from build123d import *

# Parameters (mm, degrees)
SKETCH1_W               = 49.5
SKETCH1_H               = 61.5
BOSS_EXTRUDE1_DEPTH     = 23.75
SKETCH2_W               = 46
SKETCH2_H               = 58
CUT_EXTRUDE1_DEPTH      = 22
SKETCH3_W               = 3
SKETCH3_H               = 16
CUT_EXTRUDE2_DEPTH      = 1.75
SKETCH7_W               = 3
SKETCH7_H               = 5
BOSS_EXTRUDE2_DEPTH     = 4
SKETCH11_W              = 37.5
SKETCH11_H              = 61.5
BOSS_EXTRUDE3_DEPTH     = 15
SKETCH12_W              = 34
SKETCH12_H              = 57
CUT_EXTRUDE3_DEPTH      = 15
SKETCH14_W              = 7.75
SKETCH14_H              = 9
BOSS_EXTRUDE4_DEPTH     = 3
SKETCH15_W              = 4.25
SKETCH15_H              = 5.5
CUT_EXTRUDE4_DEPTH      = 4.75
SKETCH16_W              = 8.5
SKETCH16_H              = 15.5
BOSS_EXTRUDE5_DEPTH     = 16.75
SKETCH17_W              = 5.125
SKETCH17_H              = 6.625
CUT_EXTRUDE5_DEPTH      = 8.5
CUT_EXTRUDE6_DEPTH      = 15
CUT_EXTRUDE6_DEPTH_BACK = 1.75
SKETCH18_W              = 5
SKETCH18_H              = 12
SKETCH20_W              = 16
SKETCH20_H              = 3
CUT_EXTRUDE7_DEPTH      = 1.75
SKETCH21_W              = 34.25
SKETCH21_H              = 82.5
BOSS_EXTRUDE7_DEPTH     = 10
SKETCH23_W              = 30.75
SKETCH23_H              = 79
CUT_EXTRUDE8_DEPTH      = 10
SKETCH25_W              = 3
SKETCH25_H              = 5.25
BOSS_EXTRUDE8_DEPTH     = 1.75
SKETCH28_W              = 3
SKETCH28_H              = 2
BOSS_EXTRUDE9_DEPTH     = 1.75


with BuildPart() as part:
    # Sketch1 → Boss-Extrude1 (new body)
    with BuildSketch(Plane(origin=(0, 0, 0), x_dir=(1, 0, 0), z_dir=(0, 1, 0))):
        with Locations((-113.412024913, -45.391200727)):
            Rectangle(SKETCH1_W, SKETCH1_H)
    extrude(amount=BOSS_EXTRUDE1_DEPTH)

    # Sketch2 → Cut-Extrude1 (cut)
    with BuildSketch(Plane(origin=(0, 0, 0), x_dir=(-1, 0, 0), z_dir=(0, -1, 0))):
        with Locations((113.412024913, -45.391200727)):
            Rectangle(SKETCH2_W, SKETCH2_H)
    extrude(amount=-CUT_EXTRUDE1_DEPTH, mode=Mode.SUBTRACT)

    # Sketch3 → Cut-Extrude2 (cut)
    with BuildSketch(Plane(origin=(0, 22, 0), x_dir=(-1, 0, 0), z_dir=(0, -1, 0))):
        with Locations((91.912024913, -66.391200727)):
            Rectangle(SKETCH3_W, SKETCH3_H)
        with Locations((91.912024913, -24.391200727)):
            Rectangle(SKETCH3_W, SKETCH3_H)
        with Locations((91.912024913, -45.391200727)):
            Rectangle(SKETCH3_W, SKETCH3_H)
    extrude(amount=-CUT_EXTRUDE2_DEPTH, mode=Mode.SUBTRACT)

    # Sketch7 → Boss-Extrude2 (add)
    with BuildSketch(Plane(origin=(0, 22, 0), x_dir=(-1, 0, 0), z_dir=(0, -1, 0))):
        with Locations((91.912024913, -55.891200727)):
            Rectangle(SKETCH7_W, SKETCH7_H)
        with Locations((91.912024913, -34.891200727)):
            Rectangle(SKETCH7_W, SKETCH7_H)
    extrude(amount=BOSS_EXTRUDE2_DEPTH)

    # Sketch11 → Boss-Extrude3 (add)
    with BuildSketch(Plane(origin=(0, 23.75, 0), x_dir=(1, 0, 0), z_dir=(0, 1, 0))):
        with Locations((-119.412024913, -45.391200727)):
            Rectangle(SKETCH11_W, SKETCH11_H)
    extrude(amount=BOSS_EXTRUDE3_DEPTH)

    # Sketch12 → Cut-Extrude3 (cut)
    with BuildSketch(Plane(origin=(0, 38.75, 0), x_dir=(1, 0, 0), z_dir=(0, 1, 0))):
        with Locations((-119.412024913, -45.391200727)):
            Rectangle(SKETCH12_W, SKETCH12_H)
    extrude(amount=-CUT_EXTRUDE3_DEPTH, mode=Mode.SUBTRACT)

    # Sketch14 → Boss-Extrude4 (add)
    with BuildSketch(Plane(origin=(0, 23.75, 0), x_dir=(1, 0, 0), z_dir=(0, 1, 0))):
        with Locations((-92.542024913, -66.391200727)):
            Rectangle(SKETCH14_W, SKETCH14_H)
    extrude(amount=BOSS_EXTRUDE4_DEPTH)

    # Sketch15 → Cut-Extrude4 (cut)
    with BuildSketch(Plane(origin=(0, 26.75, 0), x_dir=(1, 0, 0), z_dir=(0, 1, 0))):
        with Locations((-92.542024913, -66.391200727)):
            Rectangle(SKETCH15_W, SKETCH15_H)
    extrude(amount=-CUT_EXTRUDE4_DEPTH, mode=Mode.SUBTRACT)

    # Sketch16 → Boss-Extrude5 (add)
    with BuildSketch(Plane(origin=(0, 23.75, 0), x_dir=(1, 0, 0), z_dir=(0, 1, 0))):
        with Locations((-92.912024913, -24.391200727)):
            Rectangle(SKETCH16_W, SKETCH16_H)
    extrude(amount=BOSS_EXTRUDE5_DEPTH)

    # Sketch17 → Cut-Extrude5 (cut)
    with BuildSketch(Plane(origin=(-88.662024913, 0, 0), x_dir=(0, 0, -1), z_dir=(1, 0, 0))):
        with Locations((-27.828700727, 35.4375)):
            Rectangle(SKETCH17_W, SKETCH17_H)
        with Locations((-27.828700727, 27.0625)):
            Rectangle(SKETCH17_W, SKETCH17_H)
        with Locations((-20.953700727, 35.4375)):
            Rectangle(SKETCH17_W, SKETCH17_H)
        with Locations((-20.953700727, 27.0625)):
            Rectangle(SKETCH17_W, SKETCH17_H)
    extrude(amount=-CUT_EXTRUDE5_DEPTH, mode=Mode.SUBTRACT)

    # Sketch18 → Cut-Extrude6 (cut, two sides: drawn at the far end of the back side and taken through both)
    with BuildSketch(Plane(origin=(0, 23.75, 0), x_dir=(1, 0, 0), z_dir=(0, 1, 0)).offset(-CUT_EXTRUDE6_DEPTH_BACK)):
        with Locations((-92.912024913, -24.391200727)):
            Rectangle(SKETCH18_W, SKETCH18_H)
    extrude(amount=CUT_EXTRUDE6_DEPTH + CUT_EXTRUDE6_DEPTH_BACK, mode=Mode.SUBTRACT)

    # Sketch20 → Cut-Extrude7 (cut)
    with BuildSketch(Plane(origin=(-100.662024913, 0, 0), x_dir=(0, 0, -1), z_dir=(1, 0, 0))):
        with Locations((-45.391200727, 25.25)):
            Rectangle(SKETCH20_W, SKETCH20_H)
    extrude(amount=-CUT_EXTRUDE7_DEPTH, mode=Mode.SUBTRACT)

    # Sketch21 → Boss-Extrude7 (add)
    with BuildSketch(Plane(origin=(0, 0, 0), x_dir=(-1, 0, 0), z_dir=(0, -1, 0))):
        with Locations((153.537024913, -45.391200727)):
            Rectangle(SKETCH21_W, SKETCH21_H)
    extrude(amount=-BOSS_EXTRUDE7_DEPTH)

    # Sketch23 → Cut-Extrude8 (cut)
    with BuildSketch(Plane(origin=(0, 10, 0), x_dir=(1, 0, 0), z_dir=(0, 1, 0))):
        with Locations((-153.537024913, -45.391200727)):
            Rectangle(SKETCH23_W, SKETCH23_H)
    extrude(amount=-CUT_EXTRUDE8_DEPTH, mode=Mode.SUBTRACT)

    # Sketch25 → Boss-Extrude8 (add)
    with BuildSketch(Plane(origin=(0, 22, 0), x_dir=(-1, 0, 0), z_dir=(0, -1, 0))):
        with Locations((91.912024913, -61.016200727)):
            Rectangle(SKETCH25_W, SKETCH25_H)
        with Locations((91.912024913, -71.766200727)):
            Rectangle(SKETCH25_W, SKETCH25_H)
    extrude(amount=-BOSS_EXTRUDE8_DEPTH)

    # Sketch28 → Boss-Extrude9 (add)
    with BuildSketch(Plane(origin=(0, 23.75, 0), x_dir=(1, 0, 0), z_dir=(0, 1, 0))):
        with Locations((-91.912024913, -17.391200727)):
            Rectangle(SKETCH28_W, SKETCH28_H)
        with Locations((-91.912024913, -31.391200727)):
            Rectangle(SKETCH28_W, SKETCH28_H)
    extrude(amount=-BOSS_EXTRUDE9_DEPTH)


solid = part.part
The model under review builds one solid part; all positions refer to its coordinate system, in mm. A direction names the side the tool comes from. Round coordinates to 2 decimals unless told otherwise and drop trailing zeros. Loops run counter-clockwise (first coordinate to the right, second up) from the corner with the lowest first, then second, coordinate; pieces in that order, holes last. Notation, with made-up numbers: (-8.75, 24.5) -> (20.25, 24.5) arc R12 ccw to (20.25, 35.5) -> close; hole circle Ø1 at (-15, -24). An arc over 180 degrees is marked (long way). Write item = value, one per line. Start each with the question number.
Item 1: To check wall thickness, follow L1, parallel to X at y = 34.5, z = 32; L2, parallel to X at y = 9, z = 65.5; L3, parallel to X at y = 19, z = 71.5. State the ranges of each line that lie inside material, in increasing order.
Item 2: Take a section at C-C on y = 4.5. Give the boundary of the cut face in (x, z), plus the area to 3 significant figures.
Item 3: Mouldability with a two-part tool opening along X and no side actions: class faces 1 (the flat face through (-118, 23.75, 45)), 2 (the flat face through (-93, 32, 32.141)), 3 (the flat face through (-136.412, 5, 9)) as released by +X, released by -X, zero draft, split by the parting line, or undercut.
Item 4: Take a section at B-B on y = 34. Give the boundary of the cut face in (x, z), plus the area to 3 significant figures.
Item 5: For faces 4 (the flat face through (-120, 31, 73.891)), 5 (the flat face through (-93, 24, 63.641)), 6 (the flat face through (-93.412, 20, 35)), list the 3-axis set-ups (+Z, -Z, +X, -X, +Y, -Y) from which the entire face can be reached by the end or side of a thin tool; tool diameter is ignored.
Item 6: Take a section at A-A on z = 60.5. Give the boundary of the cut face in (x, y), plus the area to 3 significant figures.
Item 7: Take a section at D-D on x = -130.5. Give the boundary of the cut face in (y, z), plus the area to 3 significant figures.
Item 8: Insertion check: pin 1 (2 mm diameter, centred on x = -125.5, y = 22, fed in from -Z); pin 2 (1.4 mm diameter, centred on x = -89.5, z = 22, fed in from -Y); pin 3 (0.5 mm diameter, centred on x = -89, y = 27.5, fed in from +Z); pin 4 (0.9 mm diameter, centred on x = -101, z = 47.5, fed in from -Y). Each pin has a flat end and moves straight along its axis. Give the tip position at first contact, or say it passes through.
Result:
q1.L1 = -138.16 to -136.41, -102.41 to -100.66, -97.16 to -88.66
q1.L2 = -170.66 to -168.91, -138.16 to -136.41, -90.41 to -88.66
q1.L3 = -138.16 to -136.41, -90.41 to -88.66
q2.outline = (-170.66, 4.14) -> (-136.41, 4.14) -> (-136.41, 14.64) -> (-88.66, 14.64) -> (-88.66, 76.14) -> (-136.41, 76.14) -> (-136.41, 86.64) -> (-170.66, 86.64) -> close; hole (-168.91, 5.89) -> (-138.16, 5.89) -> (-138.16, 84.89) -> (-168.91, 84.89) -> close; hole (-136.41, 16.39) -> (-90.41, 16.39) -> (-90.41, 74.39) -> (-136.41, 74.39) -> close
q2.area = 665 mm²
q3.face_1 = undercut
q3.face_2 = zero draft
q3.face_3 = released by +X
q4.outline = (-138.16, 14.64) -> (-100.66, 14.64) -> (-100.66, 76.14) -> (-138.16, 76.14) -> close; (-97.16, 16.64) -> (-88.66, 16.64) -> (-88.66, 18.39) -> (-97.16, 18.39) -> close; (-97.16, 23.52) -> (-95.41, 23.52) -> (-95.41, 25.27) -> (-97.16, 25.27) -> close; (-97.16, 30.39) -> (-88.66, 30.39) -> (-88.66, 32.14) -> (-97.16, 32.14) -> close; (-90.41, 23.52) -> (-88.66, 23.52) -> (-88.66, 25.27) -> (-90.41, 25.27) -> close; hole (-136.41, 16.89) -> (-102.41, 16.89) -> (-102.41, 73.89) -> (-136.41, 73.89) -> close
q4.area = 404 mm²
q5.face_4 = +Y
q5.face_5 = +Y, -Y
q5.face_6 = -Y
q6.outline = (-170.66, 0) -> (-168.91, 0) -> (-168.91, 10) -> (-170.66, 10) -> close; (-138.16, 0) -> (-136.41, 0) -> (-136.41, 22) -> (-90.41, 22) -> (-90.41, 0) -> (-88.66, 0) -> (-88.66, 23.75) -> (-100.66, 23.75) -> (-100.66, 38.75) -> (-102.41, 38.75) -> (-102.41, 23.75) -> (-136.41, 23.75) -> (-136.41, 38.75) -> (-138.16, 38.75) -> close
q6.area = 234 mm²
q7.outline = (0, 14.64) -> (38.75, 14.64) -> (38.75, 16.89) -> (23.75, 16.89) -> (23.75, 73.89) -> (38.75, 73.89) -> (38.75, 76.14) -> (0, 76.14) -> (0, 74.39) -> (22, 74.39) -> (22, 16.39) -> (0, 16.39) -> close
q7.area = 252 mm²
q8.pin_1 = 14.64
q8.pin_2 = 0
q8.pin_3 = 32.14
q8.pin_4 = 22
